Build history of the part. All positions in model axes, mm. Face numbers are marked on the shaded views. A direction names the side the tool comes from. Round coordinates to 2 decimals unless told otherwise and drop trailing zeros. Write each loop counter-clockwise with the first axis right and the second up, starting at its lowest first coordinate (ties: lowest second). Pieces come first, ordered by that corner, then holes.
1) Saw through at A-A (x = 18). Write the cut outline in (y, z) (3 decimals), plus the area to 3 significant figures.
2) Saw through at C-C (y = 45). Write the cut outline in (x, z) (3 decimals).
3) Flat gauge pins, fed straight in: pin 1 (1.6 mm diameter, centred on x = 2.5, z = 54.5, fed in from +Y); pin 2 (5 mm diameter, centred on x = 13, y = 58.5, fed in from +Z). Where does each tip first touch, or does it go through?
4) Saw through at B-B (z = 4). Write the cut outline in (x, y) (3 decimals), plus the area to 3 significant figures.
5) Which spindle directions (+Z, -Z, +X, -X, +Y, -Y) get a long thin tool onto all of the face, cutting with end or side? Do the marked faces 5 and 6. Say none if no direction does.
6) Wall check: probe 1 along Y at (x, z) = (0, 54); probe 2 along Z at (x, y) = (21, 59.5) (3 decimals). Give the ranges that are in metal, low to high.
7) Saw through at D-D (x = 0). Write the cut outline in (y, z) (1 decimal), plus the area to 3 significant figures.
8) Pull direction Z, two halves, no side cores. Call the marked faces 1, 2, 3 and 4: +Z half, -Z half, draft (parallel to the pull), parting line (faces both ways), or undercut.
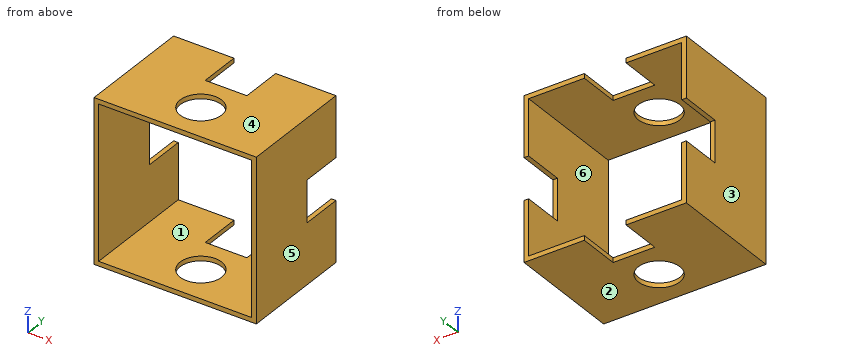
Autodesk Inventor part; units mm, degrees
ref_plane "YZ Plane" through (0, 0, 0) normal (1, 0, 0) x (0, 1, 0)
ref_plane "XZ Plane" through (0, 0, 0) normal (0, 1, 0) x (-1, 0, 0)
ref_plane "XY Plane" through (0, 0, 0) normal (0, 0, 1) x (1, 0, 0)
sketch "Sketch2" plane through (0, 0, 0) normal (0, 1, 0) x (-1, 0, 0)
  line L0 (55.88, 55.88) -> (55.88, -55.88)
  line L1 (78.232, 0) -> (-78.232, 0)
  line L2 (55.88, -55.88) -> (-55.88, -55.88)
  line L3 (-55.88, -55.88) -> (-55.88, 55.88)
  line L4 (-55.88, 55.88) -> (55.88, 55.88)
  line L5 (0, -78.232) -> (0, 78.232)
  point P0 (0, 0)
  dimension "d0" = 111.76
  dimension "d1" = 111.76
extrude "Extrusion1" add sketch "Sketch2" along normal blind 79.502
shell "Shell1" thickness 3.175 removed faces 2 at (-18.6267, 0, -18.6267) at (-18.6267, 79.502, -18.6267)
sketch "Sketch3" plane through (-55.88, 0, 55.88) normal (0, 0, 1) x (1, 0, 0)
  line L0 (111.76, 79.502) -> (0, 79.502)
  line L1 (0, 79.502) -> (41.529, 79.502)
  line L2 (41.529, 79.502) -> (41.529, 50.8)
  line L3 (41.529, 50.8) -> (70.231, 50.8)
  line L4 (70.231, 50.8) -> (70.231, 79.502)
  line L5 (70.231, 79.502) -> (41.529, 79.502)
  line L6 (108.585, 0) -> (3.175, 0)
  circle A0 centre (55.88, 25.654) radius 14.2875
  line L7 (111.76, 0) -> (111.76, 79.502)
  line L8 (0, 0) -> (0, 79.502)
  line L9 (0, 0) -> (55.88, 0)
  line L10 (55.88, 0) -> (55.88, 79.502)
  dimension "d6" = 28.702
  dimension "d10" = 28.575
  dimension "d19" = 28.702
extrude "Extrusion2" cut sketch "Sketch3" against normal up to surface (111.76 mm away) contours L4 L3 L10 L0 | L10 L3 L2 L0 | L10 A0 | A0 L10
sketch "Sketch4" plane through (55.88, 0, 55.88) normal (1, 0, 0) x (0, 0, -1)
  line L0 (0, 79.502) -> (111.76, 79.502)
  line L1 (0, 79.502) -> (41.529, 79.502)
  line L2 (41.529, 79.502) -> (41.529, 50.8)
  line L3 (41.529, 50.8) -> (70.231, 50.8)
  line L4 (70.231, 50.8) -> (70.231, 79.502)
  line L5 (70.231, 79.502) -> (41.529, 79.502)
  point P0 (55.88, 0)
  dimension "d13" = 41.529
  dimension "d14" = 28.702
  dimension "d15" = 28.702
extrude "Extrusion3" cut sketch "Sketch4" against normal up to surface (111.76 mm away)
properties part number "DIFF_HOUSING_WIP"
Evaluation:
1. outline: (0, -55.88) - (79.502, -55.88) - (79.502, -52.705) - (0, -52.705) - close; (0, 52.705) - (79.502, 52.705) - (79.502, 55.88) - (0, 55.88) - close
1. area: 505 mm2
2. outline: (-55.88, -55.88) - (55.88, -55.88) - (55.88, 55.88) - (-55.88, 55.88) - close; hole (-52.705, -52.705) - (52.705, -52.705) - (52.705, 52.705) - (-52.705, 52.705) - close
3. pin 1: stops at y = 50.8
3. pin 2: stops at z = 55.88
4. outline: (-55.88, 0) - (-52.705, 0) - (-52.705, 50.8) - (-55.88, 50.8) - close; (52.705, 0) - (55.88, 0) - (55.88, 50.8) - (52.705, 50.8) - close
4. area: 323 mm2
5. face 5: +Z, -Z, +X, +Y, -Y
5. face 6: +Y, -Y
6. probe 1: y = 0 to 11.37, 39.94 to 50.8
6. probe 2: z = -55.88 to -52.705, 52.705 to 55.88
7. outline: (0, -55.9) - (11.4, -55.9) - (11.4, -52.7) - (0, -52.7) - close; (0, 52.7) - (11.4, 52.7) - (11.4, 55.9) - (0, 55.9) - close; (39.9, -55.9) - (50.8, -55.9) - (50.8, -52.7) - (39.9, -52.7) - close; (39.9, 52.7) - (50.8, 52.7) - (50.8, 55.9) - (39.9, 55.9) - close
7. area: 141 mm2
8. face 1: undercut
8. face 2: -Z half
8. face 3: draft
8. face 4: +Z half
